Geometry: see drawing. Coordinates: mm, zero at the bounding-box minimum. A direction names the side the tool comes from. Round coordinates to 2 decimals unless told otherwise and drop trailing zeros. Loops run counter-clockwise (first coordinate to the right, second up) from the corner with the lowest first, then second, coordinate; pieces in that order, holes last. Notation, with made-up numbers: (-16.75, -7) -> (39.25, -7) arc R29 ccw to (39.25, 19) -> close; hole circle Ø9 at (8, -7). An arc over 180 degrees is marked (long way). Answer in a Markdown table with one row per item.
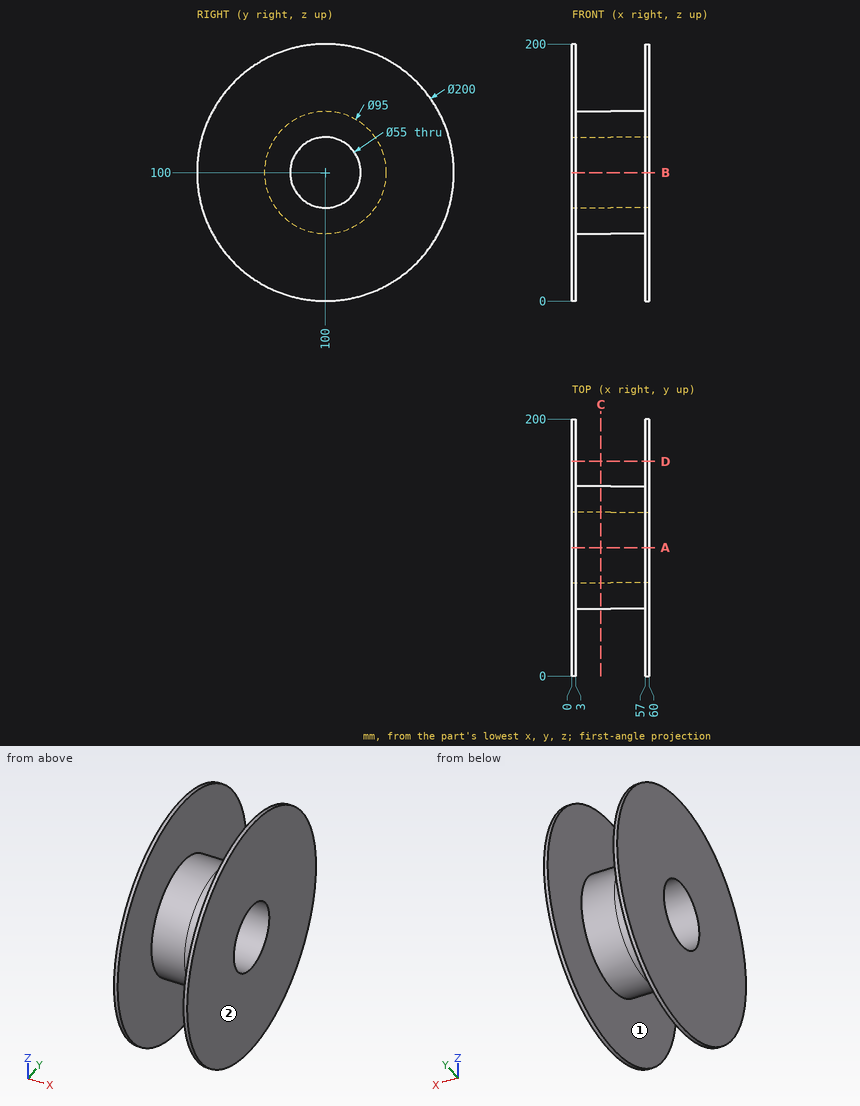
Item 1: Ray query, L1, parallel to X at y = 181.5, z = 154; L2, parallel to Z at x = 47.5, y = 100; L3, parallel to Z at x = 36, y = 119. Return the intervals inside material, ascending.
Ans:
| item | result |
|---|---|
| L1 | 0 to 3, 57 to 60 |
| L2 | 52.5 to 72.5, 127.5 to 147.5 |
| L3 | 56.47 to 80.12, 119.88 to 143.53 |
Item 2: Section query C-C, the plane x = 22.5. Output: boundary loops of the cut face in (y, z).
Ans:
| item | result |
|---|---|
| outline | circle Ø95 at (100, 100); hole circle Ø55 at (100, 100) |
Item 3: Section query D-D, the plane y = 167. Output: boundary loops of the cut face in (x, z).
Ans:
| item | result |
|---|---|
| outline | (0, 25.76) -> (3, 25.76) -> (3, 174.24) -> (0, 174.24) -> close; (57, 25.76) -> (60, 25.76) -> (60, 174.24) -> (57, 174.24) -> close |
Item 4: Section query A-A, the plane y = 100. Output: boundary loops of the cut face in (x, z), and give its area (3 significant figures).
Ans:
| item | result |
|---|---|
| outline | (0, 0) -> (3, 0) -> (3, 52.5) -> (57, 52.5) -> (57, 0) -> (60, 0) -> (60, 72.5) -> (0, 72.5) -> close; (0, 127.5) -> (60, 127.5) -> (60, 200) -> (57, 200) -> (57, 147.5) -> (3, 147.5) -> (3, 200) -> (0, 200) -> close |
| area | 3,030 mm2 |
Item 5: First-contact query: P1, Ø12, axis at x = 16.5, y = 80, coming from the +Z side; P2, Ø4, axis at x = 39, y = 89, coming from the -Z side; P3, Ø2, axis at x = 25, y = 117, coming from the +Z side. Flat tips, straight axial feed; report the tip coordinate or a pass-through.
Ans:
| item | result |
|---|---|
| P1 | z = 145.39 |
| P2 | z = 53.36 |
| P3 | z = 144.72 |
Item 6: Set-up query: the marked faces 1 and 2. Return all of +Z, -Z, +X, -X, +Y, -Y with unobstructed straight access to the full face (end or side cutting, diameter ignored); none if empty.
Ans:
| item | result |
|---|---|
| face 1 | none |
| face 2 | +Z, -Z, +X, +Y, -Y |
